Source: CAD feature listing. Evaluate the final solid. Frame: model axes, mm. Face numbers are marked on the shaded views. A direction names the side the tool comes from. Round coordinates to 2 decimals unless told otherwise and drop trailing zeros. Order: outer loops, then holes, each group sorted by start corner. A loop starts at its lowest first (then second) coordinate and runs counter-clockwise, first axis right, second up.
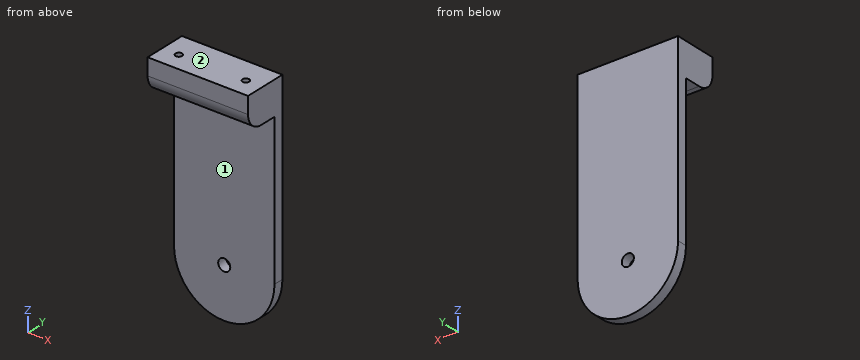
```python
from build123d import *

# Parameters (mm, degrees)
CYLINDER046_R             = 1
CYLINDER046_DEPTH         = 8
CYLINDER045_R             = 1
CYLINDER045_DEPTH         = 8
CYLINDER044_R             = 1.8
CYLINDER044_DEPTH         = 3
BOX006_W                  = 30
BOX006_H                  = 3
BOX006_DEPTH              = 55
BOX007_W                  = 30
BOX007_H                  = 10
BOX007_DEPTH              = 10
FILLET005_R               = 5
CYLINDER043_R             = 15
CYLINDER043_DEPTH         = 3
FUSION016_PLACEMENT_ANGLE = 180


with BuildPart() as arm_support_payload_plate_screw002:
    # Cylinder046 → Cylinder046 (new body)
    with BuildSketch(Plane(origin=(-10, 25, 144.7), x_dir=(1, 0, 0), z_dir=(0, 0, 1))):
        Circle(CYLINDER046_R)
    extrude(amount=CYLINDER046_DEPTH)


with BuildPart() as arm_support_payload_plate_screw001:
    # Cylinder045 → Cylinder045 (new body)
    with BuildSketch(Plane(origin=(10, 25, 144.7), x_dir=(1, 0, 0), z_dir=(0, 0, 1))):
        Circle(CYLINDER045_R)
    extrude(amount=CYLINDER045_DEPTH)


with BuildPart() as arm_support_screw_and_axis_holes:
    # Cylinder044 → Cylinder044 (new body)
    with BuildSketch(Plane(origin=(0, 32.5, 97.7), x_dir=(1, 0, 0), z_dir=(0, -1, 0))):
        Circle(CYLINDER044_R)
    extrude(amount=CYLINDER044_DEPTH)

    # Compound004: union arm-support-payload-plate-screw002, arm-support-payload-plate-screw001
    add(arm_support_payload_plate_screw002.part)
    add(arm_support_payload_plate_screw001.part)


with BuildPart() as arm_support:
    # Box006 → Box006 (new body)
    with BuildSketch(Plane(origin=(-15, -40.5, 97.7), x_dir=(1, 0, 0), z_dir=(0, 0, 1))):
        with Locations((15, 1.5)):
            Rectangle(BOX006_W, BOX006_H)
    extrude(amount=BOX006_DEPTH)


with BuildPart() as arm_screw_block_with_fillet001:
    # Box007 → Box007 (new body)
    with BuildSketch(Plane(origin=(-15, -37.5, 142.7), x_dir=(1, 0, 0), z_dir=(0, 0, 1))):
        with Locations((15, 5)):
            Rectangle(BOX007_W, BOX007_H)
    extrude(amount=BOX007_DEPTH)

    # Fillet005
    fillet005_edges = [arm_screw_block_with_fillet001.edges().sort_by_distance(p)[0] for p in [
        (0, -27.5, 142.7),
    ]]
    fillet(fillet005_edges, radius=FILLET005_R)


with BuildPart() as support_arm:
    # Cylinder043 → Cylinder043 (new body)
    with BuildSketch(Plane(origin=(0, -37.5, 97.7), x_dir=(1, 0, 0), z_dir=(0, -1, 0))):
        Circle(CYLINDER043_R)
    extrude(amount=CYLINDER043_DEPTH)

    # Fusion016: union arm-support, arm-screw-block-with-fillet001
    add(arm_support.part)
    add(arm_screw_block_with_fillet001.part)


with BuildPart() as support_arm_1:
    # Fusion016 placement: moved
    add(support_arm.part.moved(Location((0, -8, 0))).rotate(Axis((0, -8, 0), (0, 0, 1)), FUSION016_PLACEMENT_ANGLE))

    # Cut029: cut arm-support-screw-and-axis-holes
    add(arm_support_screw_and_axis_holes.part, mode=Mode.SUBTRACT)


solid = support_arm_1.part
```
1. First-contact query: pin 1 (3 mm diameter, centred on x = 2.5, y = 23, fed in from -Z); pin 2 (1.6 mm diameter, centred on x = -10, y = 24.5, fed in from +Z); pin 3 (3 mm diameter, centred on x = 7.5, z = 91.5, fed in from -Y); pin 4 (5 mm diameter, centred on y = 26, z = 106.5, fed in from -X). Flat tips, straight axial feed; report the tip coordinate or a pass-through.
2. Section C-C on x = 6.75. Return loops of the section in (y, z).
3. Access query for the marked faces 1 and 2. Directions: +Z, -Z, +X, -X, +Y, -Y. A direction counts if a zero-diameter tool reaches every point of the face in a straight line with its end or side. Return the directions, or none.
4. Line query: line 1 along Y through (x, z) = (10, 147.75); line 2 along X through (y, z) = (30.1, 97.7); line 3 along Y through (x, z) = (13.25, 132). Output: solid intervals per line, ascending.
5. Section B-B on z = 119.5. Return loops of the section in (x, y), plus the area to 3 significant figures.
6. Section D-D on y = 23. Return loops of the section in (x, z).
7. Section A-A on x = 0. Return loops of the section in (y, z), plus the area to 3 significant figures.
Result:
1. pin 1: stops at z = 142.7
1. pin 2: stops at z = 152.7
1. pin 3: stops at y = 29.5
1. pin 4: passes through
2. outline: (19.5, 147.7) arc R5 ccw to (24.5, 142.7) - (29.5, 142.7) - (29.5, 84.3) - (32.5, 84.3) - (32.5, 152.7) - (19.5, 152.7) - close
3. face 1: -Z, +X, -X, -Y
3. face 2: +Z, +X, -X, +Y, -Y
4. line 1: y = 19.5 to 24, 26 to 32.5
4. line 2: x = -15 to -1.8, 1.8 to 15
4. line 3: y = 29.5 to 32.5
5. outline: (-15, 29.5) - (15, 29.5) - (15, 32.5) - (-15, 32.5) - close
5. area: 90.0 mm2
6. outline: (-15, 142.93) - (15, 142.93) - (15, 152.7) - (-15, 152.7) - close
7. outline: (19.5, 147.7) arc R5 ccw to (24.5, 142.7) - (29.5, 142.7) - (29.5, 99.5) - (32.5, 99.5) - (32.5, 152.7) - (19.5, 152.7) - close; (29.5, 82.7) - (32.5, 82.7) - (32.5, 95.9) - (29.5, 95.9) - close
7. area: 294 mm2
